```python
from build123d import *

# Parameters (mm, degrees)
CROQUIS1_W              = 40
CROQUIS1_H              = 20
CROQUIS1_R              = 2
SALIENTE_EXTRUIR1_DEPTH = 7.5
CROQUIS2_R              = 6
CORTAR_EXTRUIR1_DEPTH   = 4
VACIADO3_T              = -1
REDONDEO1_R             = 4


with BuildPart() as part:
    # Croquis1 → Saliente-Extruir1 (new body)
    with BuildSketch(Plane(origin=(0, 0, 0), x_dir=(1, 0, 0), z_dir=(0, 1, 0))):
        Rectangle(CROQUIS1_W, CROQUIS1_H)
        with Locations(Location((-10, 0, 0), (0, 0, 270))):
            Circle(CROQUIS1_R, mode=Mode.SUBTRACT)
        with Locations(Location((10, 0, 0), (0, 0, 270))):
            Circle(CROQUIS1_R, mode=Mode.SUBTRACT)
    extrude(amount=SALIENTE_EXTRUIR1_DEPTH)

    # Croquis2 → Cortar-Extruir1 (cut)
    with BuildSketch(Plane.XZ):
        with Locations(Location((-10, 0, 0), (0, 0, 270))):
            Circle(CROQUIS2_R)
        with Locations(Location((10, 0, 0), (0, 0, 270))):
            Circle(CROQUIS2_R)
    extrude(amount=-CORTAR_EXTRUIR1_DEPTH, mode=Mode.SUBTRACT)

    # Vaciado3
    vaciado3_openings = [part.faces().sort_by_distance(p)[0] for p in [
        (0, 0, 0),
    ]]
    offset(amount=VACIADO3_T, openings=vaciado3_openings, kind=Kind.INTERSECTION)

    # Redondeo1
    redondeo1_edges = [part.edges().sort_by_distance(p)[0] for p in [
        (-19, 3.25, -9),
        (-19, 3.25, 9),
        (19, 3.25, 9),
        (19, 3.25, -9),
    ]]
    fillet(redondeo1_edges, radius=REDONDEO1_R)


solid = part.part
```
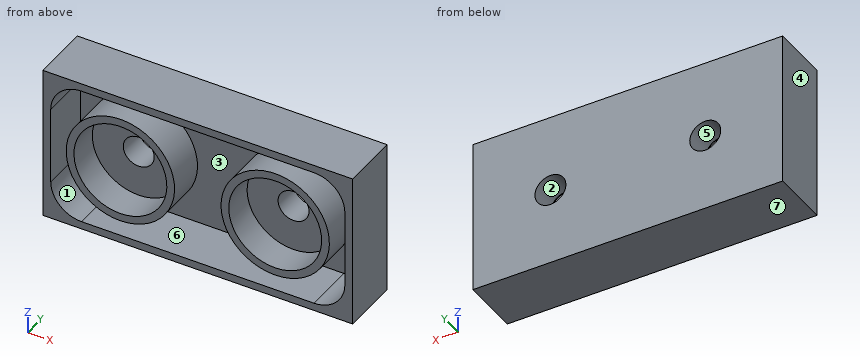
Geometry check sheet. Reference: the model listing, model coordinates, mm. Face numbers are marked on the shaded views. A direction names the side the tool comes from. Coordinates: 2 decimals unless noted, no trailing zeros. Write each loop counter-clockwise with the first axis right and the second up, starting at its lowest first coordinate (ties: lowest second). Pieces come first, ordered by that corner, then holes. Notation, with made-up numbers: (-35, -6.5) -> (-22, -6.5) arc R7 cw to (-22, 4.5) -> close; hole circle Ø2 at (-19, -28). An arc over 180 degrees is marked (long way). Use CSV: the item, a comma, the result in double quotes. Start each with the question number.
Item 1: Depth check by flat-ended pin: pin 1 Ø3.5 at (x, z) = (-10, 0) entering from -Y; pin 2 Ø2 at (x, z) = (10.5, 3) entering from -Y. Enter the tip coordinate at first touch or a pass-through.
Item 2: Cross-section at C-C, the plane z = -4. Record the cut outline in (x, y).
Item 3: Cross-section at D-D, the plane z = 8. Record the cut outline in (x, y), plus the area to 3 significant figures.
Item 4: Thickness scan on line 1 (X direction, y = 5.15, z = 0); line 2 (Z direction, x = 10, y = 5.55); line 3 (Y direction, x = -10.5, z = -4.25). Record the ranges inside material, lowest first.
Item 5: Cross-section at A-A, the plane y = 1. Record the cut outline in (x, z).
Item 6: Cross-section at B-B, the plane x = 10. Record the cut outline in (y, z).
Item 7: Mould release check, pull along X, two halves, no side actions. Record for the marked faces 4, 5, 6 and 7: released by +X, released by -X, zero draft, split by the parting line, or undercut.
Item 8: Set-up check for the marked faces 1, 2 and 3: record each of +Z, -Z, +X, -X, +Y, -Y from which the full face is reachable in a straight line by a thin tool's end or side.
Answers:
1,pin 1,"through"
1,pin 2,"y = 4"
2,outline,"(-20, 0) -> (-19, 0) -> (-19, 6.5) -> (19, 6.5) -> (19, 0) -> (20, 0) -> (20, 7.5) -> (-20, 7.5) -> close; (-15.74, 0) -> (-14.47, 0) -> (-14.47, 4) -> (-5.53, 4) -> (-5.53, 0) -> (-4.26, 0) -> (-4.26, 5) -> (-15.74, 5) -> close; (4.26, 0) -> (5.53, 0) -> (5.53, 4) -> (14.47, 4) -> (14.47, 0) -> (15.74, 0) -> (15.74, 5) -> (4.26, 5) -> close"
3,outline,"(-20, 0) -> (-17.65, 0) -> (-17.65, 6.5) -> (17.65, 6.5) -> (17.65, 0) -> (20, 0) -> (20, 7.5) -> (-20, 7.5) -> close"
3,area,"70.6 mm^2"
4,line 1,"-20 to -19, -13 to -12, -8 to -7, 7 to 8, 12 to 13, 19 to 20"
4,line 2,"-10 to -9, -3 to -2, 2 to 3, 9 to 10"
4,line 3,"4 to 5, 6.5 to 7.5"
5,outline,"(-20, -10) -> (20, -10) -> (20, 10) -> (-20, 10) -> close; circle Ø14 at (-10, 0); circle Ø14 at (10, 0); hole (-19, -5) arc R4 ccw to (-15, -9) -> (15, -9) arc R4 ccw to (19, -5) -> (19, 5) arc R4 ccw to (15, 9) -> (-15, 9) arc R4 ccw to (-19, 5) -> close; hole circle Ø12 at (-10, 0); hole circle Ø12 at (10, 0)"
6,outline,"(0, -10) -> (7.5, -10) -> (7.5, -2) -> (4, -2) -> (4, -6) -> (0, -6) -> (0, -7) -> (5, -7) -> (5, -3) -> (6.5, -3) -> (6.5, -9) -> (0, -9) -> close; (0, 6) -> (4, 6) -> (4, 2) -> (7.5, 2) -> (7.5, 10) -> (0, 10) -> (0, 9) -> (6.5, 9) -> (6.5, 3) -> (5, 3) -> (5, 7) -> (0, 7) -> close"
7,face 4,"released by -X"
7,face 5,"undercut"
7,face 6,"undercut"
7,face 7,"zero draft"
8,face 1,"-Y"
8,face 2,"+Y, -Y"
8,face 3,"none"
